Part print with two shaded views. Sizes in mm from the minimum x, y, z corner. Coordinates: 2 decimals unless noted, no trailing zeros. Loops run counter-clockwise (first coordinate to the right, second up) from the corner with the lowest first, then second, coordinate; pieces in that order, holes last.
(1) Flat gauge pins, fed straight in: P1, Ø0.8, axis at y = 5, z = 2, coming from the +X side; P2, Ø0.5, axis at y = 6, z = 2, coming from the -X side. Where does each tip first touch, or does it go through?
(2) Slice it at B-B (z = 0.7). Give the cut face in (x, y), and give its area (3 significant figures).
(3) Slice it at D-D (y = 6.75). Give the cut face in (x, z), and give its area (3 significant figures).
(4) Two-plate mould, pull along Y, no slides. Class the marked faces 1, 2, 3 and 4: pulls with the +Y half, pulls with the -Y half, needs draft (parallel to the pull), parting line crosses it, or undercut.
(5) Slice it at A-A (y = 9). Give the cut face in (x, z), and give its area (3 significant figures).
(6) Slice it at C-C (x = 13). Give the cut face in (y, z).
(7) Wall check: L1, parallel to Y at x = 13, z = 0.7; L2, parallel to X at y = 5.25, z = 1.95; L3, parallel to Z at x = 12.25, y = 4.75. Give the ranges that are in metal, low to high.
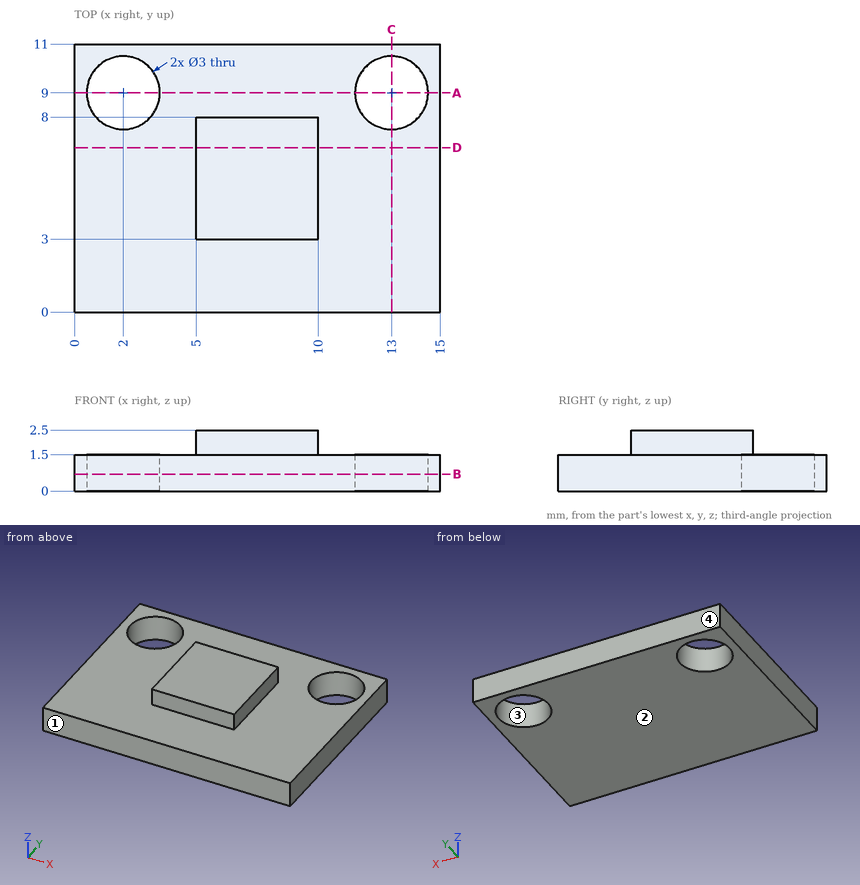
Response values:
1. P1: stops at x = 10
1. P2: stops at x = 5
2. outline: (0, 0) - (15, 0) - (15, 11) - (0, 11) - close; hole circle Ø3 at (2, 9); hole circle Ø3 at (13, 9)
2. area: 151 mm2
3. outline: (0, 0) - (15, 0) - (15, 1.5) - (10, 1.5) - (10, 2.5) - (5, 2.5) - (5, 1.5) - (0, 1.5) - close
3. area: 27.5 mm2
4. face 1: pulls with the -Y half
4. face 2: needs draft
4. face 3: undercut
4. face 4: pulls with the +Y half
5. outline: (0, 0) - (0.5, 0) - (0.5, 1.5) - (0, 1.5) - close; (3.5, 0) - (11.5, 0) - (11.5, 1.5) - (3.5, 1.5) - close; (14.5, 0) - (15, 0) - (15, 1.5) - (14.5, 1.5) - close
5. area: 13.5 mm2
6. outline: (0, 0) - (7.5, 0) - (7.5, 1.5) - (0, 1.5) - close; (10.5, 0) - (11, 0) - (11, 1.5) - (10.5, 1.5) - close
7. L1: y = 0 to 7.5, 10.5 to 11
7. L2: x = 5 to 10
7. L3: z = 0 to 1.5
